Work out the finished part from the listing and answer in its coordinate system (mm). A direction names the side the tool comes from. Give positions to 0.01 mm unless a question says otherwise; leave off trailing zeros. Order: outer loops, then holes, each group sorted by start corner. A loop starts at its lowest first (then second) coordinate and runs counter-clockwise, first axis right, second up. Notation, with made-up numbers: M 66,61 L 106,61 A10 cw 106,72 Z; hole C -4.5,58 d6. An arc over 180 degrees is marked long. One line per item, written item: value.
from build123d import *

# Parameters (mm, degrees)
SKETCH1_W           = 70
SKETCH1_H           = 70
SKETCH1_W_2         = 64
SKETCH1_H_2         = 64
BOSS_EXTRUDE1_DEPTH = 1000
FILLET1_R           = 5
SKETCH2_R           = 3
CUT_EXTRUDE1_DEPTH  = 70
SKETCH3_R           = 3
CUT_EXTRUDE2_DEPTH  = 70
LPATTERN1_COUNT     = 6
LPATTERN1_PITCH     = 35
LPATTERN1_COL_COUNT = 6
LPATTERN1_COL_PITCH = 35


with BuildPart() as part:
    # Sketch1 → Boss-Extrude1 (new body)
    with BuildSketch(Plane.XY):
        with Locations((35, 35)):
            Rectangle(SKETCH1_W, SKETCH1_H)
        with Locations((35, 35)):
            Rectangle(SKETCH1_W_2, SKETCH1_H_2, mode=Mode.SUBTRACT)
    extrude(amount=BOSS_EXTRUDE1_DEPTH)

    # Fillet1
    fillet1_edges = [part.edges().sort_by_distance(p)[0] for p in [
        (3, 67, 500),
        (3, 3, 500),
        (67, 3, 500),
        (67, 67, 500),
        (0, 70, 500),
        (70, 70, 500),
        (70, 0, 500),
        (0, 0, 500),
    ]]
    fillet(fillet1_edges, radius=FILLET1_R)

    # Sketch2 → Cut-Extrude1 (cut)
    with BuildSketch(Plane(origin=(0, 70, 0), x_dir=(1, 0, 0), z_dir=(0, 1, 0))):
        with Locations(Location((35, -965, 0), (0, 0, 270))):
            Circle(SKETCH2_R)
        with Locations(Location((35, -35, 0), (0, 0, 270))):
            Circle(SKETCH2_R)
    extrude(amount=-CUT_EXTRUDE1_DEPTH, mode=Mode.SUBTRACT)

    # Sketch3 → Cut-Extrude2 (cut)
    with BuildSketch(Plane(origin=(70, 0, 0), x_dir=(0, 0, -1), z_dir=(1, 0, 0))):
        with Locations((-500, 35)):
            Circle(SKETCH3_R)
    cut_extrude2 = extrude(amount=-CUT_EXTRUDE2_DEPTH, mode=Mode.SUBTRACT)

    # LPattern1: Cut-Extrude2 ×6
    with Locations(*[(0, 0, -i * LPATTERN1_PITCH) for i in range(1, LPATTERN1_COUNT)]):
        add(cut_extrude2, mode=Mode.SUBTRACT)

    # LPattern1 col: Cut-Extrude2 ×6
    with Locations(*[(0, 0, i * LPATTERN1_COL_PITCH) for i in range(1, LPATTERN1_COL_COUNT)]):
        add(cut_extrude2, mode=Mode.SUBTRACT)


solid = part.part
(1) Which of the six approach directions +Z, -Z, +X, -X, +Y, -Y give full straight-line access (tool end or side, diameter ignored) to faces 4 (the flat face through (35, 70, 493)), 5 (the flat face through (67, 35, 493))?
Findings:
face 4: +Z, -Z, +X, -X, +Y
face 5: +Z, -Z
(2) Section A-A, the plane x = 51 is taken. Give the vertices of the cut face in (y, z).
Findings:
outline: M 0,0 L 3,0 L 3,1000 L 0,1000 Z; M 67,0 L 70,0 L 70,1000 L 67,1000 Z
(3) Determine the mould class of faces 1 (the flat face through (70, 35, 493)), 2 (the flat face through (3, 35, 493)), 3 (the flat face through (32, 1, 0)) for opening direction X: pulls with the +X half, pulls with the -X half, needs draft (parallel to the pull), parting line crosses it, or undercut.
Findings:
face 1: pulls with the +X half
face 2: undercut
face 3: needs draft
(4) Find the intervals of material crossed by probe 1 along Y at (x, z) = (25, 165); probe 2 along Y at (x, z) = (7, 200), in increasing order. Write a range as from..to.
Findings:
probe 1: y = 0..3, 67..70
probe 2: y = 0..3.1, 66.9..70
(5) Section B-B, the plane z = 657 is taken. Give the vertices of the cut face in (x, y), then the cut area to 3 significant figures.
Findings:
outline: M 0,5 A5 ccw 5,0 L 65,0 A5 ccw 70,5 L 70,65 A5 ccw 65,70 L 5,70 A5 ccw 0,65 Z; hole M 3,8 A5 ccw 8,3 L 62,3 A5 ccw 67,8 L 67,62 A5 ccw 62,67 L 8,67 A5 ccw 3,62 Z
area: 804 mm^2
